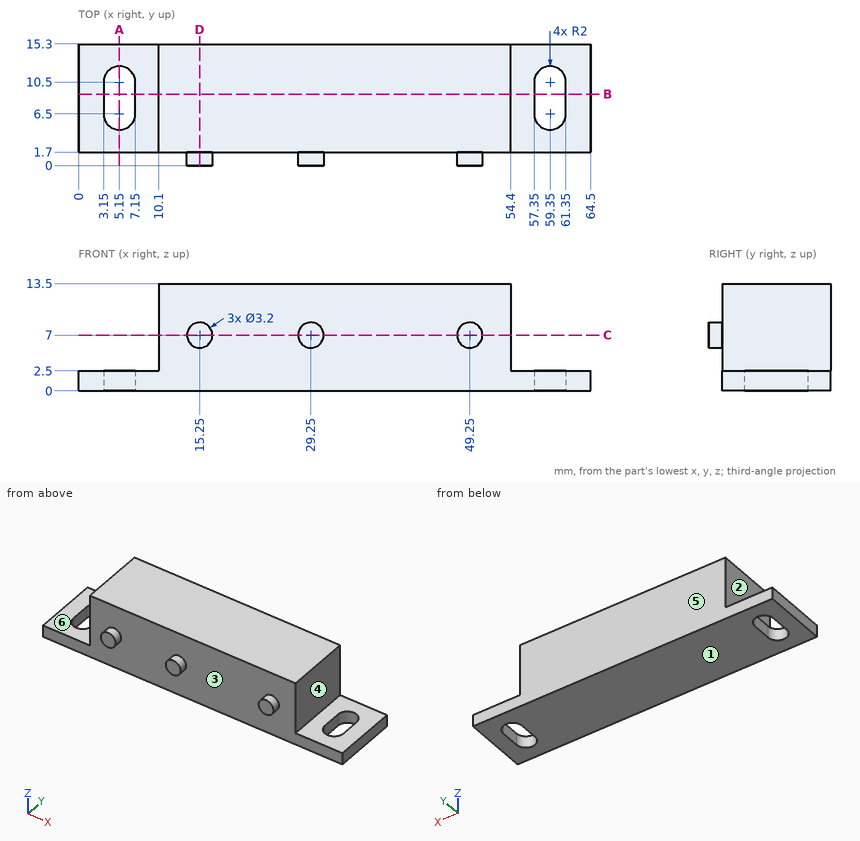
Check sheet for the drawn part. Datum: minimum x, y, z corner. Units: mm. A direction names the side the tool comes from. Give positions to 0.01 mm unless a question says otherwise; leave off trailing zeros. Loops run counter-clockwise (first coordinate to the right, second up) from the corner with the lowest first, then second, coordinate; pieces in that order, holes last.
1) Sectioned sample at A-A, the plane x = 5.15. Enter the section's corners in (y, z), then the cut area to 3 significant figures.
2) Sectioned sample at C-C, the plane z = 7. Enter the section's corners in (x, y), then the cut area to 3 significant figures.
3) Draft check along X on the marked faces 1, 2 and 3. Enter one of: pulls with the +X half, pulls with the -X half, needs draft (parallel to the pull), parting line crosses it, or undercut.
4) Depth check by flat-ended pin: pin 1 Ø5.5 at (y, z) = (10.5, 7) entering from +X; pin 2 Ø5.5 at (y, z) = (6, 5.5) entering from -X; pin 3 Ø5 at (x, y) = (58, 2.5) entering from +Z. Enter the tip coordinate at first touch or a pass-through.
5) Thickness scan on line 1 along X through (y, z) = (8, 1.25); line 2 along Y through (x, z) = (34, 8.5); line 3 along X through (y, z) = (10, 10.5). Record the ranges inside material, lowest first.
6) Set-up check for the marked faces 4, 5 and 6: record each of +Z, -Z, +X, -X, +Y, -Y from which the full face is reachable in a straight line by a thin tool's end or side.
7) Sectioned sample at B-B, the plane y = 9. Enter the section's corners in (x, z).
8) Sectioned sample at D-D, the plane x = 15.25. Enter the section's corners in (y, z).
Answers:
1. outline: (1.7, 0) - (4.5, 0) - (4.5, 2.5) - (1.7, 2.5) - close; (12.5, 0) - (15.3, 0) - (15.3, 2.5) - (12.5, 2.5) - close
1. area: 14.0 mm2
2. outline: (10.1, 1.7) - (13.65, 1.7) - (13.65, 0) - (16.85, 0) - (16.85, 1.7) - (27.65, 1.7) - (27.65, 0) - (30.85, 0) - (30.85, 1.7) - (47.65, 1.7) - (47.65, 0) - (50.85, 0) - (50.85, 1.7) - (54.4, 1.7) - (54.4, 15.3) - (10.1, 15.3) - close
2. area: 619 mm2
3. face 1: needs draft
3. face 2: pulls with the -X half
3. face 3: undercut
4. pin 1: stops at x = 54.4
4. pin 2: stops at x = 10.1
4. pin 3: stops at z = 2.5
5. line 1: x = 0 to 3.15, 7.15 to 57.35, 61.35 to 64.5
5. line 2: y = 1.7 to 15.3
5. line 3: x = 10.1 to 54.4
6. face 4: +Z, +X, +Y, -Y
6. face 5: +Z, -Z, +X, -X, +Y
6. face 6: +Z, -X, +Y, -Y
7. outline: (0, 0) - (3.15, 0) - (3.15, 2.5) - (0, 2.5) - close; (7.15, 0) - (57.35, 0) - (57.35, 2.5) - (54.4, 2.5) - (54.4, 13.5) - (10.1, 13.5) - (10.1, 2.5) - (7.15, 2.5) - close; (61.35, 0) - (64.5, 0) - (64.5, 2.5) - (61.35, 2.5) - close
8. outline: (0, 5.4) - (1.7, 5.4) - (1.7, 0) - (15.3, 0) - (15.3, 13.5) - (1.7, 13.5) - (1.7, 8.6) - (0, 8.6) - close
